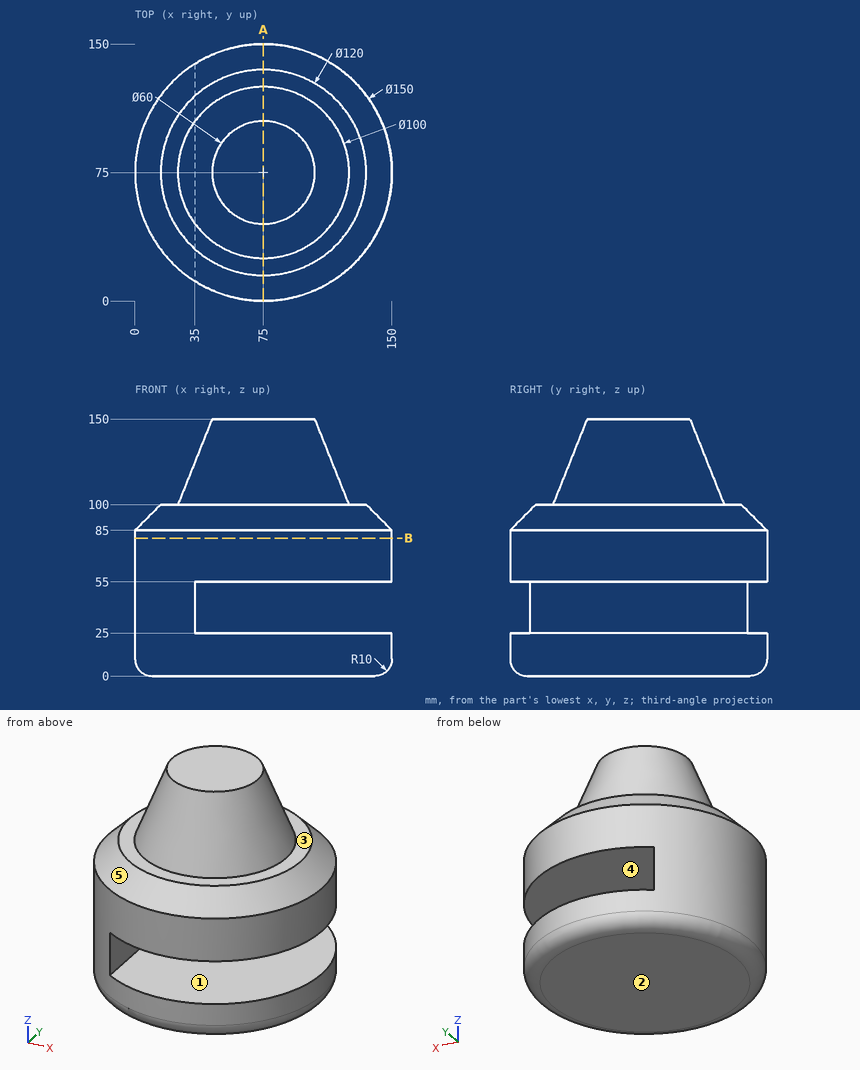
Input: dimensioned drawing with shaded views. Units: mm. Origin: part minimum x, y, z. A direction names the side the tool comes from. Round coordinates to 2 decimals unless told otherwise and drop trailing zeros. Loops run counter-clockwise (first coordinate to the right, second up) from the corner with the lowest first, then second, coordinate; pieces in that order, holes last.
1) Section query B-B on z = 80.5. Return the cut outline in (x, y).
Ans:
outline: circle Ø150 at (75, 75)
2) Pull-direction query (Z, two-part tool) for the marked faces 1, 2 and 3; classes: released by +Z, released by -Z, zero draft, split by the parting line, or undercut.
Ans:
face 1: undercut
face 2: released by -Z
face 3: released by +Z
3) Set-up query: the marked faces 4 and 5. Return all of +Z, -Z, +X, -X, +Y, -Y with unobstructed straight access to the full face (end or side cutting, diameter ignored); none if empty.
Ans:
face 4: +X, +Y, -Y
face 5: +Z
4) Section query A-A on x = 75. Return the cut outline in (y, z).
Ans:
outline: (0, 10) arc R10 ccw to (10, 0) - (140, 0) arc R10 ccw to (150, 10) - (150, 25) - (0, 25) - close; (0, 55) - (150, 55) - (150, 85) - (135, 100) - (125, 100) - (105, 150) - (45, 150) - (25, 100) - (15, 100) - (0, 85) - close
5) Pin query (flat end, axial travel): pin 1 (1 mm diameter, centred on y = 78.5, z = 115.5, fed in from -X); pin 2 (9 mm diameter, centred on y = 103.5, z = 43.5, fed in from +X); pin 3 (5 mm diameter, centred on x = 99, z = 60.5, fed in from -Y). Return the tip coordinate at first contact, or that it passes through.
Ans:
pin 1: stops at x = 31.14
pin 2: stops at x = 35
pin 3: stops at y = 3.15
6) Material intervals for line 1 (Z direction, x = 62, y = 62); line 2 (Z direction, x = 121, y = 47.5); line 3 (Z direction, x = 15.5, y = 67), sorted ascending.
Ans:
line 1: z = 0 to 25, 55 to 150
line 2: z = 0 to 25, 55 to 100
line 3: z = 0 to 99.96
